from build123d import *

# Parameters (mm, degrees)
SKETCH2_W               = 163.1
SKETCH2_H               = 171.98
SKETCH2_R               = 2.5527
SKETCH2_R_2             = 1.5875
BOSS_EXTRUDE2_DEPTH     = 1.6
FILLET1_R               = 1
CUT_EXTRUDE1_DEPTH      = 238.7151455
CUT_EXTRUDE1_DEPTH_BACK = 238.7151455
SKETCH5_R               = 1.725


with BuildPart() as part:
    # Sketch2 → Boss-Extrude2 (new body)
    with BuildSketch(Plane.XY):
        with Locations((82.55, -85.99)):
            Rectangle(SKETCH2_W, SKETCH2_H)
        with Locations((82.55, -85)):
            Circle(SKETCH2_R, mode=Mode.SUBTRACT)
        with Locations((82.55, -169.48)):
            Circle(SKETCH2_R_2, mode=Mode.SUBTRACT)
        with Locations((4.7625, -169.48)):
            Circle(SKETCH2_R_2, mode=Mode.SUBTRACT)
        with Locations((31.75, -169.48)):
            Circle(SKETCH2_R_2, mode=Mode.SUBTRACT)
        with Locations((57.15, -169.48)):
            Circle(SKETCH2_R_2, mode=Mode.SUBTRACT)
        with Locations((6.35, -94.25)):
            Circle(SKETCH2_R_2, mode=Mode.SUBTRACT)
        with Locations((6.35, -68.85)):
            Circle(SKETCH2_R_2, mode=Mode.SUBTRACT)
        with Locations((6.35, -43.45)):
            Circle(SKETCH2_R_2, mode=Mode.SUBTRACT)
        with Locations((6.35, -18.05)):
            Circle(SKETCH2_R_2, mode=Mode.SUBTRACT)
        with Locations((19.05, -3.175)):
            Circle(SKETCH2_R_2, mode=Mode.SUBTRACT)
        with Locations((44.45, -3.175)):
            Circle(SKETCH2_R_2, mode=Mode.SUBTRACT)
        with Locations((69.85, -3.175)):
            Circle(SKETCH2_R_2, mode=Mode.SUBTRACT)
        with Locations((158.75, -43.45)):
            Circle(SKETCH2_R_2, mode=Mode.SUBTRACT)
        with Locations((158.75, -18.05)):
            Circle(SKETCH2_R_2, mode=Mode.SUBTRACT)
        with Locations((146.05, -3.175)):
            Circle(SKETCH2_R_2, mode=Mode.SUBTRACT)
        with Locations((107.95, -169.48)):
            Circle(SKETCH2_R_2, mode=Mode.SUBTRACT)
        with Locations((133.35, -169.48)):
            Circle(SKETCH2_R_2, mode=Mode.SUBTRACT)
        with Locations((160.3375, -169.48)):
            Circle(SKETCH2_R_2, mode=Mode.SUBTRACT)
        with Locations((158.75, -94.25)):
            Circle(SKETCH2_R_2, mode=Mode.SUBTRACT)
        with Locations((158.75, -68.85)):
            Circle(SKETCH2_R_2, mode=Mode.SUBTRACT)
        with Locations((95.25, -3.175)):
            Circle(SKETCH2_R_2, mode=Mode.SUBTRACT)
        with Locations((120.65, -3.175)):
            Circle(SKETCH2_R_2, mode=Mode.SUBTRACT)
    extrude(amount=BOSS_EXTRUDE2_DEPTH)

    # Fillet1
    fillet1_edges = [part.edges().sort_by_distance(p)[0] for p in [
        (1, -171.98, 0.8),
        (1, 0, 0.8),
        (164.1, 0, 0.8),
        (164.1, -171.98, 0.8),
    ]]
    fillet(fillet1_edges, radius=FILLET1_R)

    # Sketch5 → Cut-Extrude1 (cut, two sides: drawn at the far end of the back side and taken through both)
    with BuildSketch(Plane.XY.offset(1.6).offset(-CUT_EXTRUDE1_DEPTH_BACK)):
        with Locations((42.775, -43.995)):
            Circle(SKETCH5_R)
        with Locations((122.325, -43.995)):
            Circle(SKETCH5_R)
        with Locations((122.325, -115.985)):
            Circle(SKETCH5_R)
        with Locations((42.775, -115.985)):
            Circle(SKETCH5_R)
    extrude(amount=CUT_EXTRUDE1_DEPTH + CUT_EXTRUDE1_DEPTH_BACK, mode=Mode.SUBTRACT)


solid = part.part
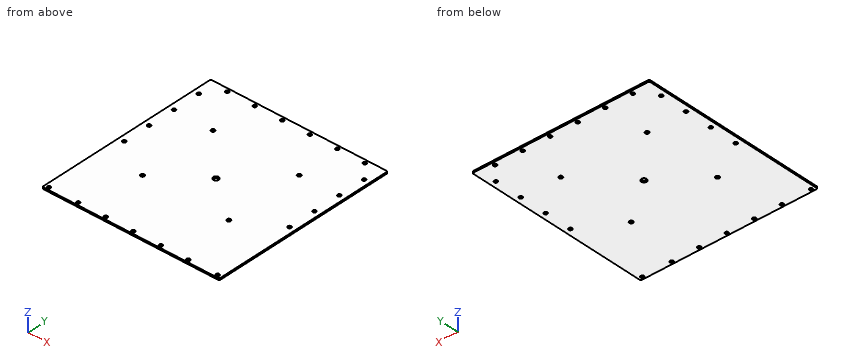
Build history of the part. All positions in model axes, mm. Give positions to 0.01 mm unless a question says otherwise; leave off trailing zeros. Loops run counter-clockwise (first coordinate to the right, second up) from the corner with the lowest first, then second, coordinate; pieces in that order, holes last. Notation, with made-up numbers: (-32.5, -1.75) -> (2.5, -1.75) arc R8 cw to (2.5, 10.25) -> close; hole circle Ø5 at (-4, -12.75). An arc over 180 degrees is marked (long way). Answer in a Markdown table with one row per item.
Item 1: Slice it at A-A on y = -85. Write the cut outline in (x, z).
Findings below:
| item | result |
|---|---|
| outline | (1, 0) -> (80, 0) -> (80, 1.6) -> (1, 1.6) -> close; (85.1, 0) -> (164.1, 0) -> (164.1, 1.6) -> (85.1, 1.6) -> close |
Item 2: Probe line 1 along X through (y, z) = (-68.85, 0.3); line 2 along Y through (x, z) = (146.05, 1.2); line 3 along X through (y, z) = (-17, 1.45). List the from-to ranges inside material, lowest first. Write a range as [from, to].
Findings below:
| item | result |
|---|---|
| line 1 | x = [1, 4.76], [7.94, 157.16], [160.34, 164.1] |
| line 2 | y = [-171.98, -4.76], [-1.59, 0] |
| line 3 | x = [1, 5.16], [7.54, 157.56], [159.94, 164.1] |
Item 3: Flat gauge pin, fed straight in: P1, Ø1.9, axis at x = 158.75, y = -18.05, coming from the -Z side. Where does the tip first touch, or does it go through?
Findings below:
| item | result |
|---|---|
| P1 | passes through |
